```python
from build123d import *

# Parameters (mm, degrees)
CROQUIS1_R              = 75
CROQUIS1_R_2            = 5.5
SALIENTE_EXTRUIR2_DEPTH = 90
SALIENTE_EXTRUIR3_DEPTH = 20
CROQUIS3_R              = 12.677450178
CORTAR_EXTRUIR1_DEPTH   = 110
CROQUIS7_R              = 86.720907706
CROQUIS7_R_2            = 31.991589163
CORTAR_EXTRUIR6_DEPTH   = 42
SALIENTE_EXTRUIR5_START = -40
CROQUIS8_R              = 12.677450178
SALIENTE_EXTRUIR5_DEPTH = 40


with BuildPart() as part:
    # Croquis1 → Saliente-Extruir2 (new body)
    with BuildSketch(Plane.XY):
        with Locations(Location((-0.300298633, -0.001591846, 0), (0, 0, 180))):
            Circle(CROQUIS1_R)
        with Locations(Location((38.084343476, 38.301334696, 0), (0, 0, 180))):
            Circle(CROQUIS1_R_2, mode=Mode.SUBTRACT)
        with Locations(Location((53.921710963, -0.069731009, 0), (0, 0, 180))):
            Circle(CROQUIS1_R_2, mode=Mode.SUBTRACT)
        with Locations(Location((38.017275671, -38.400881717, 0), (0, 0, 180))):
            Circle(CROQUIS1_R_2, mode=Mode.SUBTRACT)
        with Locations(Location((-0.383085558, -54.238249204, 0), (0, 0, 180))):
            Circle(CROQUIS1_R_2, mode=Mode.SUBTRACT)
        with Locations(Location((-38.714236265, -38.304518389, 0), (0, 0, 180))):
            Circle(CROQUIS1_R_2, mode=Mode.SUBTRACT)
        with Locations(Location((-54.551603752, 0.066547317, 0), (0, 0, 180))):
            Circle(CROQUIS1_R_2, mode=Mode.SUBTRACT)
        with Locations(Location((-38.617872937, 38.397698024, 0), (0, 0, 180))):
            Circle(CROQUIS1_R_2, mode=Mode.SUBTRACT)
        with Locations(Location((-0.246807232, 54.235065511, 0), (0, 0, 180))):
            Circle(CROQUIS1_R_2, mode=Mode.SUBTRACT)
    extrude(amount=SALIENTE_EXTRUIR2_DEPTH)

    # Croquis2 → Saliente-Extruir3 (add)
    with BuildSketch(Plane(origin=(0, 0, 0), x_dir=(-1, 0, 0), z_dir=(0, 0, -1))):
        with BuildLine():
            Line((26.112208604, 38.727030057), (27.485456967, 53.179425602))
            ThreePointArc((27.485456967, 53.179425602), (24.429171845, 58.268515598), (18.664650888, 56.850766019))
            Line((18.664650888, 56.850766019), (9.322520199, 45.625098372))
            ThreePointArc((9.322520199, 45.625098372), (0.246807232, 41.725065511), (-8.828905735, 45.625098372))
            Line((-8.828905735, 45.625098372), (-18.077259399, 56.815518496))
            ThreePointArc((-18.077259399, 56.815518496), (-24.061995546, 57.38682812), (-26.914903807, 52.094912031))
            Line((-26.914903807, 52.094912031), (-25.583042051, 37.551282353))
            ThreePointArc((-25.583042051, 37.551282353), (-29.618728772, 29.072115687), (-38.414038327, 25.78189313))
            Line((-38.414038327, 25.78189313), (-52.866433872, 27.155141493))
            ThreePointArc((-52.866433872, 27.155141493), (-57.489082017, 23.336218016), (-55.768515975, 17.592290361))
            Line((-55.768515975, 17.592290361), (-45.299902018, 9.018464332))
            ThreePointArc((-45.299902018, 9.018464332), (-41.406181734, 0.471020463), (-44.548158548, -8.380410835))
            Line((-44.548158548, -8.380410835), (-55.738578672, -17.628764499))
            ThreePointArc((-55.738578672, -17.628764499), (-57.481280164, -23.378316923), (-52.860896821, -27.218423606))
            Line((-52.860896821, -27.218423606), (-37.951986277, -25.85311053))
            ThreePointArc((-37.951986277, -25.85311053), (-29.390923032, -29.288425153), (-25.491911386, -37.648502822))
            Line((-25.491911386, -37.648502822), (-26.86515975, -52.100898367))
            ThreePointArc((-26.86515975, -52.100898367), (-24.027008592, -57.407327586), (-18.034758099, -56.853949712))
            Line((-18.034758099, -56.853949712), (-8.692627409, -45.628282064))
            ThreePointArc((-8.692627409, -45.628282064), (0.383085558, -41.728249204), (9.458798525, -45.628282064))
            Line((9.458798525, -45.628282064), (18.707152189, -56.818702189))
            ThreePointArc((18.707152189, -56.818702189), (24.46680217, -58.2561123), (27.540433688, -53.177480099))
            Line((27.540433688, -53.177480099), (26.208571932, -38.633850421))
            ThreePointArc((26.208571932, -38.633850421), (29.868330432, -29.458612556), (39.043568298, -25.798854055))
            Line((39.043568298, -25.798854055), (53.495963843, -27.172102419))
            ThreePointArc((53.495963843, -27.172102419), (58.58505384, -24.115817297), (57.16730426, -18.35129634))
            Line((57.16730426, -18.35129634), (45.941636613, -9.00916565))
            ThreePointArc((45.941636613, -9.00916565), (42.041603752, 0.066547317), (45.941636613, 9.142260284))
            Line((45.941636613, 9.142260284), (57.132056737, 18.390613948))
            ThreePointArc((57.132056737, 18.390613948), (58.569466849, 24.150263929), (53.490834648, 27.223895446))
            Line((53.490834648, 27.223895446), (38.94720497, 25.892033691))
            ThreePointArc((38.94720497, 25.892033691), (29.771967104, 29.551792191), (26.112208604, 38.727030057))
        make_face()
    extrude(amount=SALIENTE_EXTRUIR3_DEPTH)

    # Croquis3 → Cortar-Extruir1 (cut)
    with BuildSketch(Plane(origin=(0, 0, -20), x_dir=(-1, 0, 0), z_dir=(0, 0, -1))):
        Circle(CROQUIS3_R)
    extrude(amount=-CORTAR_EXTRUIR1_DEPTH, mode=Mode.SUBTRACT)

    # Croquis7 → Cortar-Extruir6 (cut)
    with BuildSketch(Plane.XY.offset(90)):
        Circle(CROQUIS7_R)
        Circle(CROQUIS7_R_2, mode=Mode.SUBTRACT)
    extrude(amount=-CORTAR_EXTRUIR6_DEPTH, mode=Mode.SUBTRACT)

    # Croquis8 → Saliente-Extruir5 (add)
    with BuildSketch(Plane.XY.offset(90).offset(SALIENTE_EXTRUIR5_START)):
        with Locations(Location((0, 0, 0), (0, 0, 180))):
            Circle(CROQUIS8_R)
        with BuildLine():
            Line((4.407319519, 4.947589036), (-4.407319519, 4.947589036))
            ThreePointArc((-4.407319519, 4.947589036), (0, -6.62594164), (4.407319519, 4.947589036))
        make_face(mode=Mode.SUBTRACT)
    extrude(amount=SALIENTE_EXTRUIR5_DEPTH)


solid = part.part
```
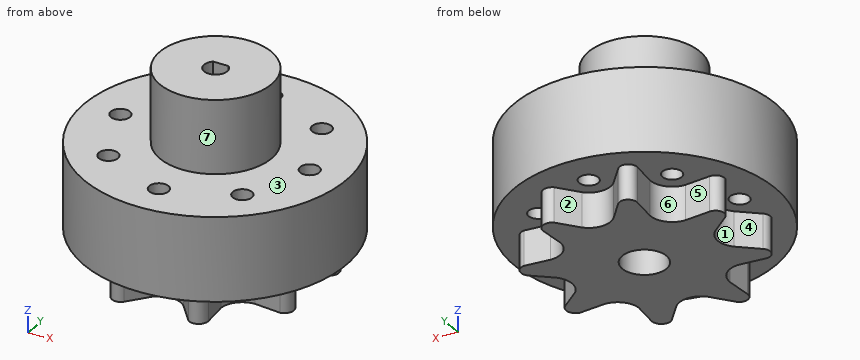
Check sheet for the modelled part. Datum: model origin and axes. Units: mm. Face numbers are marked on the shaded views. A direction names the side the tool comes from. Round coordinates to 2 decimals unless told otherwise and drop trailing zeros. Order: outer loops, then holes, each group sorted by start corner. A loop starts at its lowest first (then second) coordinate and runs counter-clockwise, first axis right, second up. Notation, with made-up numbers: (87.5, 2) -> (116.5, 2) arc R14 cw to (116.5, 18) -> close; hole circle Ø10 at (73, 83.5). An arc over 180 degrees is marked (long way). One line per item, written item: value. Start each with the question number.
Q1. Cross-section at A-A (x = 0). Record the boundary of the cut face in (y, z), and give its area (3 significant figures).
Q2. Mould release check, pull along X, two halves, no side actions. Record for the marked faces 4, 5, 6 and 7: pulls with the +X half, pulls with the -X half, needs draft (parallel to the pull), parting line crosses it, or undercut.
Q3. Cross-section at D-D (x = 15.5). Record the boundary of the cut face in (y, z), and give its area (3 significant figures).
Q4. Gauge pin test, flat ends, axial feed: pin 1 Ø10 at (y, z) = (-35.5, 45) entering from -X; pin 2 Ø4 at (x, y) = (-47.5, -6) entering from +Z; pin 3 Ø17.5 at (x, y) = (-54.55, 0.07) entering from -Z. Record the tip position at first contact, or that the pin passes through.
Q5. Thickness scan on line 1 (X direction, y = 0, z = 2); line 2 (Y direction, x = 0, z = 80); line 3 (X direction, y = -38.5, z = 7.5). Record the ranges inside material, lowest first.
Q6. Cross-section at B-B (z = 22.5). Give the number of separate pieces and of enclosed holes in the cut face, and give its area (3 significant figures).
Q7. Set-up check for the marked faces 1, 2 and 3: record each of +Z, -Z, +X, -X, +Y, -Y from which the full face is reachable in a straight line by a thin tool's end or side.
Q8. Cross-section at C-C (z = 55). Record the boundary of the cut face in (x, y).
Completed:
1. outline: (-75, 0) -> (-59.72, 0) -> (-59.72, 48) -> (-75, 48) -> close; (-48.75, 0) -> (-41.73, 0) -> (-41.73, -20) -> (-12.68, -20) -> (-12.68, 50) -> (-6.63, 50) -> (-6.63, 90) -> (-31.99, 90) -> (-31.99, 48) -> (-48.75, 48) -> close; (4.95, 50) -> (12.68, 50) -> (12.68, -20) -> (41.73, -20) -> (41.73, 0) -> (48.74, 0) -> (48.74, 48) -> (31.99, 48) -> (31.99, 90) -> (4.95, 90) -> close; (59.73, 0) -> (75, 0) -> (75, 48) -> (59.73, 48) -> close
1. area: 8,260 mm²
2. face 4: pulls with the -X half
2. face 5: undercut
2. face 6: undercut
2. face 7: parting line crosses it
3. outline: (-73.32, 0) -> (-53.81, 0) -> (-53.81, -20) -> (53.7, -20) -> (53.7, 0) -> (73.32, 0) -> (73.32, 48) -> (27.99, 48) -> (27.99, 90) -> (-27.99, 90) -> (-27.99, 48) -> (-73.32, 48) -> close
3. area: 11,500 mm²
4. pin 1: stops at x = -68.82
4. pin 2: stops at z = 48
4. pin 3: stops at z = 0
5. line 1: x = -75.3 to -60.05, -49.05 to -12.68, 12.68 to 48.42, 59.42 to 74.7
5. line 2: y = -31.99 to -6.63, 4.95 to 31.99
5. line 3: x = -64.67 to -44.21, -33.22 to 32.52, 43.52 to 64.06
6. separate pieces: 1
6. enclosed holes: 9
6. area: 16,400 mm²
7. face 1: -Z, -X
7. face 2: -Z, +Y
7. face 3: +Z
8. outline: circle Ø63.98 at (0, 0); hole (-4.41, 4.95) arc R6.63 ccw (long way) to (4.41, 4.95) -> close
